The model under review builds one solid part; all positions refer to its coordinate system, in mm. Face numbers are marked on the shaded views. A direction names the side the tool comes from. Round coordinates to 2 decimals unless told otherwise and drop trailing zeros. Order: outer loops, then holes, each group sorted by start corner. A loop starts at its lowest first (then second) coordinate and runs counter-clockwise, first axis right, second up. Notation, with made-up numbers: M 71,64 L 76,64 A30 ccw 76,88 Z; hole C -2.5,-7 d7. An arc over 180 degrees is marked long. Answer as a JSON object with one key per item and string values. Group by question number.
1. Machinability: for the marked faces 4 and 5, which of the approach directions +Z, -Z, +X, -X, +Y, -Y give a long, thin tool a straight path to every point of the face, cutting with its end or side? Answer none if there is none.
2. Add section C-C on y = -2.75. State the section outline as (x, z) points, and give its area (3 significant figures).
3. Add section A-A on z = 8. State the section outline as (x, y) points, and give its area (3 significant figures).
4. Mouldability with a two-part tool opening along X and no side actions: class the marked faces 1, 2 and 3 as released by +X, released by -X, zero draft, split by the parting line, or undercut.
5. To check wall thickness, follow probe 1 along Y at (x, z) = (0, 9); probe 2 along Y at (x, z) = (-1.75, 34.5); probe 3 along X at (y, z) = (3, 14). State the ranges of each line that lie inside material, in increasing order. Write a range as [from, to].
6. Clearance check with flat-ended pins moving along their axes: P1, Ø4, axis at x = 2.5, y = 4, coming from the -Z side; P2, Ø1.5, axis at y = -4, z = 11, coming from the +X side; P3, Ø3, axis at x = 4, z = 16.5, coming from the +Y side; P4, Ø6, axis at y = 4, z = 18, coming from the +X side. State where each tip first meets the part, or that it passes through.
7. Add section B-B on x = -3.25. State the section outline as (y, z) points, and give its area (3 significant figures).
```python
from build123d import *

# Parameters (mm, degrees)
SKETCH1_R                 = 7.07
BOSS_EXTRUDE1_DEPTH       = 40
M5X0_8_TAPPED_HOLE1_D     = 4.2
M5X0_8_TAPPED_HOLE1_DEPTH = 12.4
M5X0_8_TAPPED_HOLE1_TIP   = 1.2618073
M5X0_8_TAPPED_HOLE3_D     = 4.2
M5X0_8_TAPPED_HOLE3_DEPTH = 12.4
M5X0_8_TAPPED_HOLE3_TIP   = 1.2618073


with BuildPart() as part:
    # Sketch1 → Boss-Extrude1 (new body)
    with BuildSketch(Plane(origin=(0, 0, 0), x_dir=(0, 1, 0), z_dir=(0, 0, 1))):
        with Locations(Location((0, 0, 0), (0, 0, 270))):
            Circle(SKETCH1_R)
    extrude(amount=BOSS_EXTRUDE1_DEPTH)

    # M5x0.8 Tapped Hole1
    with Locations(Plane.XY.offset(40)):
        with Locations((0, 0)):
            Hole(M5X0_8_TAPPED_HOLE1_D / 2, depth=M5X0_8_TAPPED_HOLE1_DEPTH)
            with Locations((0, 0, -(M5X0_8_TAPPED_HOLE1_DEPTH + M5X0_8_TAPPED_HOLE1_TIP / 2))):  # 118° drill point
                Cone(0, M5X0_8_TAPPED_HOLE1_D / 2, M5X0_8_TAPPED_HOLE1_TIP, mode=Mode.SUBTRACT)

    # M5x0.8 Tapped Hole3
    with Locations(Plane(origin=(0, 0, 0), x_dir=(-1, 0, 0), z_dir=(0, 0, -1))):
        with Locations((0, 0)):
            Hole(M5X0_8_TAPPED_HOLE3_D / 2, depth=M5X0_8_TAPPED_HOLE3_DEPTH)
            with Locations((0, 0, -(M5X0_8_TAPPED_HOLE3_DEPTH + M5X0_8_TAPPED_HOLE3_TIP / 2))):  # 118° drill point
                Cone(0, M5X0_8_TAPPED_HOLE3_D / 2, M5X0_8_TAPPED_HOLE3_TIP, mode=Mode.SUBTRACT)


solid = part.part
```
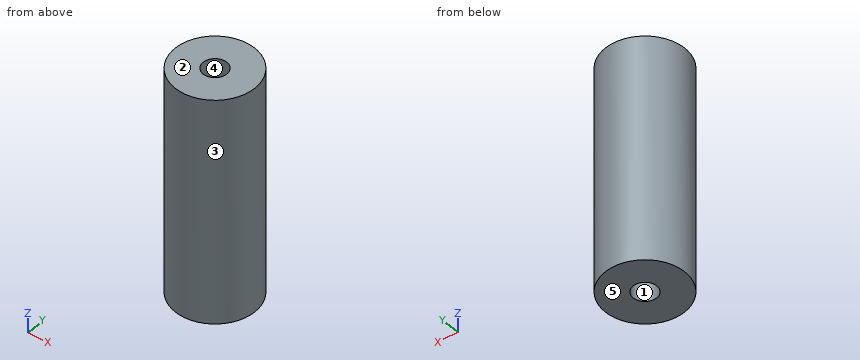
Recorded:
{
 "1": {"face 4": "+Z", "face 5": "-Z, +X, -X, +Y, -Y"},
 "2": {"outline": "M -6.51,0 L 6.51,0 L 6.51,40 L -6.51,40 Z", "area": "521 mm²"},
 "3": {"outline": "C 0,0 d14.14; hole C 0,0 d4.2", "area": "143 mm²"},
 "4": {"face 1": "undercut", "face 2": "zero draft", "face 3": "split by the parting line"},
 "5": {"probe 1": "y = [-7.07, -2.1], [2.1, 7.07]", "probe 2": "y = [-6.85, -1.16], [1.16, 6.85]", "probe 3": "x = [-6.4, 6.4]"},
 "6": {"P1": "stops at z = 0", "P2": "stops at x = 6.28", "P3": "stops at y = 6.61", "P4": "stops at x = 7"},
 "7": {"outline": "M -6.28,0 L 6.28,0 L 6.28,40 L -6.28,40 Z", "area": "502 mm²"}
}
